from build123d import *

# Parameters (mm, degrees)
SKETCH2_R           = 24
BOSS_EXTRUDE1_DEPTH = 19.916428128
SKETCH3_R           = 1.25
CUT_EXTRUDE1_DEPTH  = 40.353070007
SKETCH4_R           = 1.6
CUT_EXTRUDE2_DEPTH  = 40.353070007
SKETCH5_R           = 0.5
CUT_EXTRUDE3_DEPTH  = 39.148813636


# Read off the part's stored shape, not the designer's step: Roller coating 12, Roller core 12 coated
with BuildPart() as part:
    # Roller coating 12 outline → Roller coating 12 (revolve)
    with BuildSketch(Plane.YX):
        with BuildLine():
            ThreePointArc((12.7, -17.916428128), (15.217989764, 0), (12.7, 17.916428128))
            Line((12.7, 17.916428128), (8, 17.916428128))
            Line((8, 17.916428128), (8, 17.416428128))
            Line((8, 17.416428128), (12.322080058, 17.416428128))
            ThreePointArc((12.322080058, 17.416428128), (14.717989764, 0), (12.322080058, -17.416428128))
            Line((12.322080058, -17.416428128), (8, -17.416428128))
            Line((8, -17.416428128), (8, -17.916428128))
            Line((8, -17.916428128), (12.7, -17.916428128))
        make_face()
    revolve(axis=Axis((0, 0, 0), (1, 0, 0)))


with BuildPart() as body_2:
    # Roller core 12 coated outline → Roller core 12 coated (revolve)
    with BuildSketch(Plane.YX):
        with BuildLine():
            Line((1.25, 17.416428128), (1.25, -17.416428128))
            Line((1.25, -17.416428128), (12.322080058, -17.416428128))
            ThreePointArc((12.322080058, -17.416428128), (14.717989764, 0), (12.322080058, 17.416428128))
            Line((12.322080058, 17.416428128), (1.25, 17.416428128))
        make_face()
    revolve(axis=Axis((0, 0, 0), (1, 0, 0)))


with BuildPart() as part_1:
    add(part.part)

    # Combine1: union body 2
    add(body_2.part)


with BuildPart() as body_2_2:
    # Sketch2 → Boss-Extrude1 (new body)
    with BuildSketch(Plane(origin=(0, 0, 0), x_dir=(0, 0, -1), z_dir=(1, 0, 0))):
        Circle(SKETCH2_R)
    extrude(amount=-BOSS_EXTRUDE1_DEPTH)

    # Combine2: cut part
    add(part_1.part, mode=Mode.SUBTRACT)

    # Sketch3 → Cut-Extrude1 (cut, through all)
    with BuildSketch(Plane(origin=(0, 0, 0), x_dir=(0, 0, -1), z_dir=(1, 0, 0))):
        Circle(SKETCH3_R)
    extrude(amount=-CUT_EXTRUDE1_DEPTH, mode=Mode.SUBTRACT)

    # Sketch4 → Cut-Extrude2 (cut, through all)
    with BuildSketch(Plane(origin=(0, 0, 0), x_dir=(0, 0, -1), z_dir=(1, 0, 0))):
        with Locations((0, 19.608994882)):
            Circle(SKETCH4_R)
        with Locations((-19.608994882, 0)):
            Circle(SKETCH4_R)
        with Locations((0, -19.608994882)):
            Circle(SKETCH4_R)
        with Locations((19.608994882, 0)):
            Circle(SKETCH4_R)
    extrude(amount=-CUT_EXTRUDE2_DEPTH, mode=Mode.SUBTRACT)

    # Sketch5 → Cut-Extrude3 (cut, through all)
    with BuildSketch(Plane(origin=(-17.416428128, 0, 0), x_dir=(0, 0, -1), z_dir=(1, 0, 0))):
        with Locations((-7.071067812, 7.071067812)):
            Circle(SKETCH5_R)
        with Locations((0, 10)):
            Circle(SKETCH5_R)
        with Locations((-10, 0)):
            Circle(SKETCH5_R)
        with Locations((0, -10)):
            Circle(SKETCH5_R)
        with Locations((10, 0)):
            Circle(SKETCH5_R)
        with Locations((7.071067812, 7.071067812)):
            Circle(SKETCH5_R)
        with Locations((-7.071067812, -7.071067812)):
            Circle(SKETCH5_R)
        with Locations((7.071067812, -7.071067812)):
            Circle(SKETCH5_R)
    extrude(amount=-CUT_EXTRUDE3_DEPTH, mode=Mode.SUBTRACT)


solid = body_2_2.part
Check sheet for the modelled part. Datum: model origin and axes. Units: mm. A direction names the side the tool comes from. Give positions to 0.01 mm unless a question says otherwise; leave off trailing zeros. Order: outer loops, then holes, each group sorted by start corner. A loop starts at its lowest first (then second) coordinate and runs counter-clockwise, first axis right, second up. Notation, with made-up numbers: M -29,5 L 26,5 A11 cw 26,24 Z; hole C -13,67 d1. An arc over 180 degrees is marked long. Answer as CSV lines item,"result". Start each with the question number.
Item 1: Cross-section at A-A on z = 20. Enter the section's corners in (x, y).
Item 2: Thickness scan on line 1 (Y direction, x = -19.35, z = 0); line 2 (X direction, y = -9.5, z = -2); line 3 (Y direction, x = -2.75, z = -19.5). Record the ranges inside material, lowest first. Write a range as [from, to].
Item 3: Mould release check, pull along Z, two halves, no side actions. Record for faces 3 (the face through (-9.819, 18.047, 0.347)), 4 (the face through (-9.819, 1.055, 23.977)), 5 (the face through (0, 11, 11)): +Z half, -Z half, draft (parallel to the pull), parting line (faces both ways), or undercut.
Item 4: Tool access check on faces 1 (the face through (-18.65, 0.38, -1.19)), 2 (the face through (-17.67, -1.73, -7.81)). Record the directions out of +Z, -Z, +X, -X, +Y, -Y that give a thin tool (end or side, any length) a straight path to the whole face; none if there is none.
Item 5: Cross-section at B-B on x = -1.75. State how many separate pieces and enclosed holes the cut face has, plus the area to 3 significant figures.
Item 6: Gauge pin test, flat ends, axial feed: P1, Ø12.5, axis at y = -2, z = 5, coming from the +X side; P2, Ø1, axis at x = -9, y = -2, coming from the +Z side; P3, Ø10, axis at x = -11.5, z = 11, coming from the +Y side. Record the tip position at first contact, or that the pin passes through.
Established:
1,outline,"M -19.92,-13.27 L 0,-13.27 L 0,-1.55 L -19.92,-1.55 Z; M -19.92,1.55 L 0,1.55 L 0,13.27 L -19.92,13.27 Z"
2,line 1,"y = [-24, -21.21], [-18.01, -10.5], [-9.5, -1.25], [1.25, 9.5], [10.5, 18.01], [21.21, 24]"
2,line 2,"x = [-19.92, -17.92]"
2,line 3,"y = [-13.99, -1.6], [1.6, 13.99]"
3,face 3,"undercut"
3,face 4,"parting line"
3,face 5,"draft"
4,face 1,"+X, -X"
4,face 2,"+X"
5,separate pieces,"1"
5,enclosed holes,"5"
5,area,"1,050 mm^2"
6,P1,"stops at x = -17.42"
6,P2,"stops at z = 23.95"
6,P3,"stops at y = 23.24"
